```python
from build123d import *

# Parameters (mm, degrees)
F0_R     = 11
F1_DEPTH = 7


with BuildPart() as f1:
    # F0 (on Top) → F1 (new body)
    with BuildSketch(Plane.XY):
        with BuildLine():
            ThreePointArc((18.15895, 36), (-1e-06, 54.158951), (-18.158952, 36))
            Line((-18.158952, 36), (-18.158952, -36))
            ThreePointArc((-18.158952, -36), (-1e-06, -54.158951), (18.15895, -36))
            Line((18.15895, -36), (18.15895, 36))
        make_face()
        with Locations((-1e-06, -36)):
            Circle(F0_R, mode=Mode.SUBTRACT)
        with Locations((-1e-06, 36)):
            Circle(F0_R, mode=Mode.SUBTRACT)
        Circle(F0_R, mode=Mode.SUBTRACT)
    extrude(amount=F1_DEPTH)


solid = f1.part
```
Check sheet for the modelled part. Datum: model origin and axes. Units: mm. Round coordinates to 2 decimals unless told otherwise and drop trailing zeros. Order: outer loops, then holes, each group sorted by start corner. A loop starts at its lowest first (then second) coordinate and runs counter-clockwise, first axis right, second up.
1) Section check D-D (x = 6.5). Record the boundary of the cut face in (y, z).
2) Scan lines: line 1 (Y direction, x = 0, z = 2); line 2 (Y direction, x = -8, z = 5.25); line 3 (Y direction, x = 15, z = 4). Record each from-to range of solid material in increasing order.
3) Section check A-A (z = 4.75). Record the boundary of the cut face in (x, y).
4) Section check C-C (y = 0). Record the boundary of the cut face in (x, z), and give its area (3 significant figures).
5) Section check B-B (x = 0). Record the boundary of the cut face in (y, z), and give its area (3 significant figures).
6) Mould release check, pull along Y, two halves, no side actions. Record for faces 1 (the cylindrical face through (-0.399, -54.155, 3.451)), 2 (the cylindrical face through (0.399, 54.155, 3.451)), 3 (the flat face through (0, 13, 0)), 4 (the cylindrical face through (-1.432, 46.906, 3.451)): +Y half, -Y half, draft (parallel to the pull), parting line (faces both ways), or undercut.
Result:
1. outline: (-52.96, 0) - (-44.87, 0) - (-44.87, 7) - (-52.96, 7) - close; (-27.13, 0) - (-8.87, 0) - (-8.87, 7) - (-27.13, 7) - close; (8.87, 0) - (27.13, 0) - (27.13, 7) - (8.87, 7) - close; (44.87, 0) - (52.96, 0) - (52.96, 7) - (44.87, 7) - close
2. line 1: y = -54.16 to -47, -25 to -11, 11 to 25, 47 to 54.16
2. line 2: y = -52.3 to -43.55, -28.45 to -7.55, 7.55 to 28.45, 43.55 to 52.3
2. line 3: y = -46.23 to 46.23
3. outline: (-18.16, -36) arc R18.16 ccw to (18.16, -36) - (18.16, 36) arc R18.16 ccw to (-18.16, 36) - close; hole circle Ø22 at (0, -36); hole circle Ø22 at (0, 0); hole circle Ø22 at (0, 36)
4. outline: (-18.16, 0) - (-11, 0) - (-11, 7) - (-18.16, 7) - close; (11, 0) - (18.16, 0) - (18.16, 7) - (11, 7) - close
4. area: 100 mm2
5. outline: (-54.16, 0) - (-47, 0) - (-47, 7) - (-54.16, 7) - close; (-25, 0) - (-11, 0) - (-11, 7) - (-25, 7) - close; (11, 0) - (25, 0) - (25, 7) - (11, 7) - close; (47, 0) - (54.16, 0) - (54.16, 7) - (47, 7) - close
5. area: 296 mm2
6. face 1: -Y half
6. face 2: +Y half
6. face 3: draft
6. face 4: undercut
